from build123d import *

# Parameters (mm, degrees)
F1_DEPTH = 56.75
F2_R     = 4
F4_DEPTH = 7
F5_R     = 1
F6_R     = 2


with BuildPart() as f1:
    # F0 (on Front) → F1 (new body, symmetric)
    with BuildSketch(Plane.XZ):
        Polygon((47.2216577835, 0), (51.2216577835, 0), (51.2216577835, 50.8734804946), (50.37642126, 52.6860960687), (-52.4895125687, 4.7189233611), (-51.2216577835, 2), (-51.2216577835, 0), (-47.2216577835, 0), (-47.2216577835, 2.8867786506), (-47.1738083736, 2.7841652599), (47.2216577835, 46.8014940241), align=None)
    extrude(amount=F1_DEPTH, both=True)

    # F2
    f2_edges = [f1.edges().sort_by_distance(p)[0] for p in [
        (51.221658, 0, 50.87348),
        (-51.221658, 0, 2),
    ]]
    fillet(f2_edges, radius=F2_R)

    # F3 (on face) → F4 (join)
    with BuildSketch(Plane(origin=(-11.1824046347, 0, 23.980744127), x_dir=(0.906307787, 0, 0.4226182617), z_dir=(-0.4226182617, 0, 0.906307787))):
        with BuildLine():
            Line((6.0774126859, -12.25), (14.5774126859, -12.25))
            ThreePointArc((14.5774126859, -12.25), (15.2845194671, -11.9571067812), (15.5774126859, -11.25))
            Line((15.5774126859, -11.25), (15.5774126859, 11.25))
            ThreePointArc((15.5774126859, 11.25), (15.2845194671, 11.9571067812), (14.5774126859, 12.25))
            Line((14.5774126859, 12.25), (6.0774126859, 12.25))
            ThreePointArc((6.0774126859, 12.25), (5.3703059047, 11.9571067812), (5.0774126859, 11.25))
            Line((5.0774126859, 11.25), (5.0774126859, -11.25))
            ThreePointArc((5.0774126859, -11.25), (5.3703059047, -11.9571067812), (6.0774126859, -12.25))
        make_face()
    extrude(amount=F4_DEPTH)

    # F5
    f5_edges = [f1.edges().sort_by_distance(p)[0] for p in [
        (-4.780918, -12.25, 34.689452),
    ]]
    fillet(f5_edges, radius=F5_R)

    # F6
    f6_edges = [f1.edges().sort_by_distance(p)[0] for p in [
        (51.221658, -56.75, 24.993351),
        (51.221658, 56.75, 24.993351),
    ]]
    fillet(f6_edges, radius=F6_R)


solid = f1.part
Read the model definition and answer for the solid it produces. Units are mm, in the model's axes. A direction names the side the tool comes from. Give positions to 0.01 mm unless a question says otherwise; leave off trailing zeros. Write each loop counter-clockwise with the first axis right and the second up, starting at its lowest first coordinate (ties: lowest second). Pieces come first, ordered by that corner, then holes. Notation, with made-up numbers: M -15.5,-14.5 L -4.5,-14.5 A6 cw -4.5,-6.5 Z; hole C 3,58 d9. An arc over 180 degrees is marked long. One line per item, written item: value. Start each with the question number.
(1) Determine the mould class of faces 1 (the flat face through (51.222, -1, 25)), 2 (the flat face through (-7.83, 0.16, 28.81)), 3 (the cylindrical face through (-4.6, -12, 34.4)) for opening direction Z: pulls with the +Z half, pulls with the -Z half, needs draft (parallel to the pull), parting line crosses it, or undercut.
(2) Find section C-C (x = 20.5). Determine the outline of the cut face in (y, z), plus the area to 3 significant figures.
(3) Find section B-B (z = 13). Determine the outline of the cut face in (x, y), plus the area to 3 significant figures.
(4) Flat-ended cylindrical pins translate along their axes: pin 1 Ø4 at (x, y) = (17, -41.5) entering from -Z; pin 2 Ø12 at (y, z) = (-16, 15) entering from -X; pin 3 Ø12 at (x, y) = (-38, -36) entering from -Z. Find the tip coordinate at first contact, or state that the pin passes through.
(5) Find the intervals of material crossed by line 1 (X direction, y = 43, z = 28.5); line 2 (X direction, y = -19.5, z = 37.5); line 3 (Z direction, x = -39.5, y = 45), in increasing order.
(6) A tool of negligible diameter and unlimited length cuts with its end or side. For faces 4 (the flat face through (1.685, -0.157, 33.245)), 5 (the cylindrical face through (1.43, 11.95, 33.12)), 6 (the flat face through (47.222, -1, 24)), from which of +Z, -Z, +X, -X, +Y, -Y can it reach the whole face along a straight path? Write none if from no direction.
(7) Find section A-A (y = -32). Determine the outline of the cut face in (x, z), plus the area to 3 significant figures.
Results below:
1. face 1: needs draft
1. face 2: undercut
1. face 3: pulls with the +Z half
2. outline: M -56.75,34.34 L 56.75,34.34 L 56.75,38.75 L -56.75,38.75 Z
2. area: 501 mm^2
3. outline: M -34.73,-56.75 L -25.27,-56.75 L -25.27,56.75 L -34.73,56.75 Z; M 47.22,-56.75 L 49.22,-56.75 A2 ccw 51.22,-54.75 L 51.22,54.75 A2 ccw 49.22,56.75 L 47.22,56.75 Z
3. area: 1,530 mm^2
4. pin 1: stops at z = 31.78
4. pin 2: stops at x = -43.31
4. pin 3: stops at z = 4.26
5. line 1: x = -1.49 to 7.97, 47.22 to 51.22
5. line 2: x = 17.81 to 27.27, 47.22 to 51.22
5. line 3: z = 6.36 to 10.78
6. face 4: +Z, +Y, -Y
6. face 5: +Z, +Y
6. face 6: -Z, +Y, -Y
7. outline: M -52.49,4.72 L -51.6,2.8 A4 cw -51.22,1.11 L -51.22,0 L -47.22,0 L -47.22,2.89 L -47.17,2.78 L 47.22,46.8 L 47.22,0 L 51.22,0 L 51.22,49.99 A4 ccw 50.85,51.68 L 50.38,52.69 Z
7. area: 652 mm^2
